Could you check a few things on this model? Use its own coordinates, in mm. A direction names the side the tool comes from. Round coordinates to 2 decimals unless told otherwise and drop trailing zeros. Loops run counter-clockwise (first coordinate to the right, second up) from the corner with the lowest first, then second, coordinate; pieces in that order, holes last. Notation, with made-up numbers: (38, 13) -> (75, 13) arc R20 cw to (75, 33) -> close; hole circle Ø4 at (-22.75, 41). An arc over 180 degrees is marked (long way). One line per item, written item: value.
```python
from build123d import *

# Parameters (mm, degrees)
SKETCH1_R           = 1.75
SKETCH1_R_2         = 5
BOSS_EXTRUDE1_DEPTH = 10
EXTRUDE1_DEPTH      = 5
FILLET2_R           = 20
FILLET3_R           = 5
FILLET5_R           = 5
EXTRUDE2_DEPTH      = 5
FILLET7_R           = 475
FILLET8_R           = 15
FILLET9_R           = 5
SKETCH4_R           = 3.5
EXTRUDE3_DEPTH      = 1


with BuildPart() as part:
    # Sketch1 → Boss-Extrude1 (new body)
    with BuildSketch(Plane.XY):
        with BuildLine():
            Line((59.115327383, 43.551262968), (93.822811009, 43.551262968))
            ThreePointArc((93.822811009, 43.551262968), (97.822811009, 39.551262968), (93.822811009, 35.551262968))
            Line((93.822811009, 35.551262968), (73.221068218, 35.551262968))
            ThreePointArc((73.221068218, 35.551262968), (65.430500205, 30.870379763), (65.905746743, 21.794160382))
            add(Edge.make_bspline(
                [(65.905746743, 21.794160382), (68.510586107, 17.931817085), (68.397648351, 12.955422289), (67.785956814, 7.945306105)],
                knots=[0, 0, 0, 0, 1, 1, 1, 1], degree=3))
            ThreePointArc((67.785956814, 7.945306105), (67.117243875, 5.990433735), (65.715264602, 4.47281814))
            ThreePointArc((65.715264602, 4.47281814), (62.263505272, 3.582643734), (59.096031047, 5.217929635))
            ThreePointArc((59.096031047, 5.217929635), (55.724954026, 7.67997226), (51.642471122, 8.551262968))
            Line((51.642471122, 8.551262968), (46.626949913, 8.551262968))
            ThreePointArc((46.626949913, 8.551262968), (39.555882101, 11.480195156), (36.626949913, 18.551262968))
            Line((36.626949913, 18.551262968), (36.626949913, 38.848632096))
            ThreePointArc((36.626949913, 38.848632096), (42.251881835, 47.568318218), (52.515088487, 46.03881686))
            ThreePointArc((52.515088487, 46.03881686), (55.588605185, 44.19379373), (59.115327383, 43.551262968))
        make_face()
        with Locations((93.822811009, 39.551262968)):
            Circle(SKETCH1_R, mode=Mode.SUBTRACT)
        with Locations((62.822811009, 39.551262968)):
            Circle(SKETCH1_R, mode=Mode.SUBTRACT)
        with Locations((62.822811009, 8.551262968)):
            Circle(SKETCH1_R, mode=Mode.SUBTRACT)
        with Locations((45.725055781, 39.551262968)):
            Circle(SKETCH1_R_2, mode=Mode.SUBTRACT)
        with Locations((45.725055781, 17.551264875)):
            Circle(SKETCH1_R_2, mode=Mode.SUBTRACT)
    extrude(amount=-BOSS_EXTRUDE1_DEPTH)

    # Sketch2 → Extrude1 (add)
    with BuildSketch(Plane.XY):
        Polygon((45.636633265, 8.551262968), (43.896905309, 0.551262968), (13.896905309, 0.551262968), (13.896905309, 16.551262968), (39.149006125, 16.551262968), (41.006428166, 12.551262968), (45.636633265, 10.857586925), align=None)
    extrude(amount=-EXTRUDE1_DEPTH)

    # Fillet2
    # the kernel refuses this fillet: 20 mm, written as the material it adds along each edge
    with BuildSketch(Plane(origin=(36.828990942, 16.551262968, -5), x_dir=(-0.010101536018348446, 0.9999489781834221, 0), z_dir=(0, 0, 1))) as fillet2_piece_1:
        with BuildLine():
            CenterArc((20.203051209, 19.998979564), FILLET2_R, 179.421214776, 90)
            Line((0.204071645, 20.201010284), (-1.795826311, 20.221213356))
            Line((-1.795826311, 20.221213356), (-1.999897956, 0.020203072))
            Line((-1.999897956, 0.020203072), (0.380184704, -1.963532427))
            ThreePointArc((0.380184704, -1.963532427), (1.981735809, -1.818070308), (19.980817416, -1.999897956))
            Line((19.980817416, -1.999897956), (20.001020488, 0))
        make_face()
    extrude(amount=5)

    # Fillet3
    fillet3_edges = [part.edges().sort_by_distance(p)[0] for p in [
        (13.896905309, 16.551262968, -2.5),
    ]]
    fillet(fillet3_edges, radius=FILLET3_R)

    # Fillet5
    fillet5_edges = [part.edges().sort_by_distance(p)[0] for p in [
        (13.896905309, 0.551262968, -2.5),
    ]]
    fillet(fillet5_edges, radius=FILLET5_R)

    # Sketch3 → Extrude2 (cut)
    with BuildSketch(Plane(origin=(0, 0, -5), x_dir=(-1, 0, 0), z_dir=(0, 0, -1))):
        with BuildLine():
            Line((-17.230767467, 10.918134064), (-35.230767467, 10.918134064))
            ThreePointArc((-35.230767467, 10.918134064), (-36.730767467, 12.418134064), (-35.230767467, 13.918134064))
            Line((-35.230767467, 13.918134064), (-17.230767467, 13.918134064))
            ThreePointArc((-17.230767467, 13.918134064), (-15.730767467, 12.418134064), (-17.230767467, 10.918134064))
        make_face()
        with BuildLine():
            Line((-17.225055781, 2.918134064), (-40.725055781, 2.918134064))
            ThreePointArc((-40.725055781, 2.918134064), (-42.225055781, 4.418134064), (-40.725055781, 5.918134064))
            Line((-40.725055781, 5.918134064), (-17.225055781, 5.918134064))
            ThreePointArc((-17.225055781, 5.918134064), (-15.725055781, 4.418134064), (-17.225055781, 2.918134064))
        make_face()
    extrude(amount=-EXTRUDE2_DEPTH, mode=Mode.SUBTRACT)

    # Fillet7
    # the kernel refuses this fillet: 475 mm, written as the material it adds along each edge
    with BuildSketch(Plane(origin=(45.636633265, 8.600420143, -5), x_dir=(0, -1, 0), z_dir=(0, 0, 1))) as fillet7_piece_1:
        with BuildLine():
            CenterArc((475.04890177, 0.492579304), FILLET7_R, 179.941199476, 0.118216777)
            ThreePointArc((0.049151908, 0.980054022), (0.036604611, 0.489423747), (0, 0))
            Line((0, 0), (0.049157175, 0))
        make_face()
    extrude(amount=5)

    # Fillet8
    # the kernel refuses this fillet: 15 mm, written as the material it adds along each edge
    with BuildSketch(Plane(origin=(45.636633265, 8.551262968, 0), x_dir=(0.999999999985564, 5.37325013854713e-06, 0), z_dir=(0, 0, -1))) as fillet8_piece_1:
        with BuildLine():
            CenterArc((13.580951994, 8.137405625), FILLET8_R, 192.269167845, 20.584390422)
            Line((-1.076449047, 4.949836848), (0, 0))
            ThreePointArc((0, 0), (0.490027011, -0.000252765), (0.980054022, 0))
        make_face()
    extrude(amount=5)

    # Fillet9
    fillet9_edges = [part.edges().sort_by_distance(p)[0] for p in [
        (43.896905309, 0.551262968, -2.5),
    ]]
    fillet(fillet9_edges, radius=FILLET9_R)

    # Sketch4 → Extrude3 (cut)
    with BuildSketch(Plane(origin=(0, 0, -10), x_dir=(-1, 0, 0), z_dir=(0, 0, -1))):
        with Locations((-62.822811009, 39.551262968)):
            Circle(SKETCH4_R)
        with Locations((-93.822811009, 39.551262968)):
            Circle(SKETCH4_R)
        with Locations((-62.822811009, 8.551262968)):
            Circle(SKETCH4_R)
    extrude(amount=-EXTRUDE3_DEPTH, mode=Mode.SUBTRACT)


solid = part.part
```
(1) For pin 1 Ø4 at (x, z) = (32.5, -3) entering from +Y; pin 2 Ø1 at (x, z) = (72.5, -6) entering from +Y; pin 3 Ø5 at (y, z) = (31.5, -4.5) entering from -X, each with a flat end and sliding along its axis, tell me the tip position at first contact or that it passes through.
Results below:
pin 1: stops at y = 27.58
pin 2: stops at y = 43.55
pin 3: stops at x = 35.15
(2) Imagine slicing it at C-C on y = 32. Write out the boundary of the cut face in (x, z).
Results below:
outline: (36.1, -5) -> (36.63, -5) -> (36.63, -10) -> (66.15, -10) -> (66.15, 0) -> (36.1, 0) -> close
(3) Please list where these lines run through material, in increasing order: L1, parallel to X at y = 5, z = -2.75; L2, parallel to Y at x = 45, z = -7; L3, parallel to Y at x = 24.5, z = -2.
Results below:
L1: x = 13.93 to 15.84, 42.11 to 44.94, 59.3 to 66.34
L2: y = 8.68 to 12.6, 22.5 to 34.6, 44.5 to 48.34
L3: y = 0.55 to 2.92, 5.92 to 10.92, 13.92 to 18.17
(4) On a 3-axis mill with a long thin cutter (end or side, diameter ignored), from which of +Z, -Z, +X, -X, +Y, -Y can I reach the whole of each face in a straight line? I mean faces 4 (the face through (36.627, 29, -7)), 5 (the face through (29, 5.918, -3)), 6 (the face through (61, 38, -9)). Say none if no direction works.
Results below:
face 4: -Z, -X, +Y
face 5: +Z, -Z
face 6: -Z
(5) Imagine slicing it at B-B on z = -3.25. Give the number of separate pieces and of enclosed holes in the cut face, then the cut area to 3 significant figures.
Results below:
separate pieces: 1
enclosed holes: 7
area: 1,580 mm²
(6) Imagine slicing it at A-A on x = 86. Write out the boundary of the cut face in (y, z), then the cut area to 3 significant figures.
Results below:
outline: (35.55, -10) -> (43.55, -10) -> (43.55, 0) -> (35.55, 0) -> close
area: 80.0 mm²
(7) We'd pull the mould along X, two halves only. Please class faces 1 (the face through (42.1, 47.5, -4.9)), 2 (the face through (41.757, 14.509, -4.93)), 3 (the face through (47, 24, 0)): +X half, -X half, draft (parallel to the pull), parting line (faces both ways), or undercut.
Results below:
face 1: parting line
face 2: undercut
face 3: draft
